Verification items for the finished model (mm, model axes). A direction names the side the tool comes from. Coordinates: 2 decimals unless noted, no trailing zeros. Order: outer loops, then holes, each group sorted by start corner. A loop starts at its lowest first (then second) coordinate and runs counter-clockwise, first axis right, second up. Notation, with made-up numbers: (59, 43) -> (78, 43) arc R19 cw to (78, 79) -> close; hole circle Ø3 at (57.5, 29). An arc over 180 degrees is marked (long way). Use CSV: the item, a comma, the result in double quotes. Start each with the question number.
1) Sectioned sample at B-B on y = 147.5. Record the boundary of the cut face in (x, z).
2) Sectioned sample at A-A on z = -7. Record the boundary of the cut face in (x, y), then the cut area to 3 significant figures.
3) Go/stop test with flat-tipped pins: pin 1 (12 mm diameter, centred on x = 15.5, z = 23.5, fed in from +Y); pin 2 (8 mm diameter, centred on x = 0, z = 32.5, fed in from +Y); pin 3 (4 mm diameter, centred on x = 0, z = -32.5, fed in from +Y). Record where each tip stops, or that it passes through.
4) Sectioned sample at C-C on x = 17. Record the boundary of the cut face in (y, z), then the cut area to 3 significant figures.
5) Scan lines: line 1 along Z through (x, y) = (0, 232); line 2 along Y through (x, z) = (-18.5, 36). Record each from-to range of solid material in increasing order.
6) Tool access check on faces 1 (the flat face through (11.5, 243, -5.9)), 2 (the flat face through (0, 289.5, 0)). Record the directions out of +Z, -Z, +X, -X, +Y, -Y that give a thin tool (end or side, any length) a straight path to the whole face; none if there is none.
7) Release check for a two-part mould opening along X. For faces 3 (the cylindrical face through (-30.1, 232.6, -0.53)), 4 (the cylindrical face through (-8.43, 269.22, -4.38)), 5 (the flat face through (1, 0, 1)) record: released by +X, released by -X, zero draft, split by the parting line, or undercut.
Solid Edge part; units mm, degrees
sketch "Sketch1" plane through (0, 0, 0) normal (0, -1, 0) x (1, 0, 0)
  circle A0 centre (0, 0) radius 41
extrude "Protrusion1" add sketch "Sketch1" against normal blind 136.5
sketch "Sketch2" plane through (0, 136.5, 0) normal (0, 1, 0) x (0, 0, -1)
  circle A0 centre (0, 0) radius 41
extrude "Stufenzahl_3" add sketch "Sketch2" along normal blind 103.2
sketch "Sketch3" plane through (0, 239.7, 0) normal (0, 1, 0) x (0, 0, -1)
  circle A0 centre (0, 0) radius 25
extrude "Extrusionsausprägung_3" add sketch "Sketch3" along normal blind 3.3
sketch "Sketch4" plane through (0, 243, 0) normal (0, 1, 0) x (0, 0, -1)
  circle A0 centre (0, 0) radius 12.5
extrude "Extrusionsausprägung_4" add sketch "Sketch4" along normal blind 6.5
sketch "Sketch5" plane through (0, 249.5, 0) normal (0, 1, 0) x (0, 0, -1)
  circle A0 centre (0, 0) radius 9.5
extrude "Extrusionsausprägung_5" add sketch "Sketch5" along normal blind 40
hole "Bohrung_1" at (0, 239.7, -32.5) direction (0, -1, 0) diameter 4.917 depth 14 tip angle 118 thread major 6 thread length 10
hole "Hole1" at (-32.5, 239.7, 0) direction (0, -1, 0) diameter 4.917 depth 14 tip angle 118 thread major 6 thread length 10
hole "Hole2" at (0, 239.7, 32.5) direction (0, -1, 0) diameter 4.917 depth 14 tip angle 118 thread major 6 thread length 10
hole "Hole3" at (32.5, 239.7, 0) direction (0, -1, 0) diameter 4.917 depth 14 tip angle 118 thread major 6 thread length 10
Answers follow:
1,outline,"circle Ø82 at (0, 0)"
2,outline,"(-40.4, 0) -> (40.4, 0) -> (40.4, 239.7) -> (24, 239.7) -> (24, 243) -> (10.36, 243) -> (10.36, 249.5) -> (6.42, 249.5) -> (6.42, 289.5) -> (-6.42, 289.5) -> (-6.42, 249.5) -> (-10.36, 249.5) -> (-10.36, 243) -> (-24, 243) -> (-24, 239.7) -> (-40.4, 239.7) -> close"
2,area,"20,200 mm²"
3,pin 1,"stops at y = 243"
3,pin 2,"stops at y = 239.7"
3,pin 3,"stops at y = 225.42"
4,outline,"(0, -37.31) -> (239.7, -37.31) -> (239.7, -18.33) -> (243, -18.33) -> (243, 18.33) -> (239.7, 18.33) -> (239.7, 37.31) -> (0, 37.31) -> close"
4,area,"18,000 mm²"
5,line 1,"z = -41 to -34.96, -30.04 to 30.04, 34.96 to 41"
5,line 2,"y = 0 to 239.7"
6,face 1,"+Y"
6,face 2,"+Z, -Z, +X, -X, +Y"
7,face 3,"undercut"
7,face 4,"split by the parting line"
7,face 5,"zero draft"
